Input: part model. Units: mm. Frame: model coordinates. A direction names the side the tool comes from. Coordinates: 2 decimals unless noted, no trailing zeros. Write each loop counter-clockwise with the first axis right and the second up, starting at its lowest first coordinate (ties: lowest second). Pieces come first, ordered by that corner, then holes. Notation, with made-up numbers: (-35.75, 19) -> (-31.75, 19) arc R29 ccw to (-31.75, 50) -> close; hole circle Ø4 at (-15, -31.5). An arc over 180 degrees is marked (long way). Use one line per item in the form item = value. Start each with the question number.
(1) Set-up query: faces 1 (the face through (-51, -7.62, 3)), 2 (the face through (-0.486, -91.437, 0.715)), 3 (the face through (13, -25, 3.175)). Return all of +Z, -Z, +X, -X, +Y, -Y with unobstructed straight access to the full face (end or side cutting, diameter ignored); none if empty.
(2) Pull-direction query (Y, two-part tool) for faces 4 (the face through (13, 19, 3.175)), 5 (the face through (-69.85, 0, 1)), 6 (the face through (-68.604, 32.175, 0.715)); classes: released by +Y, released by -Y, zero draft, split by the parting line, or undercut.
(3) Cut plane B-B on x = 12.7. State how many separate pieces and enclosed holes the cut face has, plus the area to 3 significant figures.
(4) Cut plane A-A on y = 0. Return the cut outline in (x, z) (3 decimals).
(5) First-contact query: pin 1 (3 mm diameter, centred on x = -44.5, y = 1, fed in from -Z); pin 2 (9 mm diameter, centred on x = -25.4, y = 0, fed in from -Z) (3 decimals); pin 3 (5 mm diameter, centred on x = -18, z = 3, fed in from +Y). Flat tips, straight axial feed; report the tip coordinate or a pass-through.
(6) Ray query, line 1 along Y through (x, z) = (0, 2) (3 decimals); line 2 along Y through (x, z) = (12.5, 2.25); line 3 along Z through (x, y) = (-30.5, 22). Return the intervals inside material, ascending.
(7) Cut plane C-C on y = -50.8. Return the cut outline in (x, z) (3 decimals), plus the area to 3 significant figures.
```python
from build123d import *

# Parameters (mm, degrees)
F2_R     = 2.3876
F2_R_2   = 2.794
F2_R_3   = 1.3
F3_DEPTH = 6.35
F4_R     = 6.5
F5_DEPTH = 3.175
F7_DEPTH = 5.08
F8_R     = 15.875
F9_DEPTH = 25.4


with BuildPart() as f3:
    # F2 (on Top) → F3 (new body)
    with BuildSketch(Plane.XY):
        with BuildLine():
            ThreePointArc((30.6280254128, -77.5120508256), (38.0547799414, -65.063355973), (40.64, -50.8))
            ThreePointArc((40.64, -50.8), (-14.263355973, -12.7452200586), (-30.6280254128, -77.5120508256))
            ThreePointArc((-30.6280254128, -77.5120508256), (0, -91.44), (30.6280254128, -77.5120508256))
        make_face()
        with Locations((-28.596158833, -67.31)):
            Circle(F2_R, mode=Mode.SUBTRACT)
        with Locations((28.596158833, -67.31)):
            Circle(F2_R, mode=Mode.SUBTRACT)
        with Locations((0, -17.78)):
            Circle(F2_R, mode=Mode.SUBTRACT)
        with Locations((12.7, -21.9970452561)):
            Circle(F2_R_2, mode=Mode.SUBTRACT)
        with BuildLine():
            ThreePointArc((-30.6280254128, -77.5120508256), (-14.263355973, -12.7452200586), (40.64, -50.8))
            ThreePointArc((40.64, -50.8), (38.0547799414, -65.063355973), (30.6280254128, -77.5120508256))
            Line((30.6280254128, -77.5120508256), (65.1568869123, -37.9212738245))
            ThreePointArc((65.1568869123, -37.9212738245), (68.6381780975, -32.0859481123), (69.85, -25.4))
            Line((69.85, -25.4), (69.85, 25.4))
            ThreePointArc((69.85, 25.4), (68.6381780975, 32.0859481123), (65.1568869123, 37.9212738245))
            Line((65.1568869123, 37.9212738245), (30.6280254128, 77.5120508256))
            ThreePointArc((30.6280254128, 77.5120508256), (38.0547799414, 65.063355973), (40.64, 50.8))
            ThreePointArc((40.64, 50.8), (-14.263355973, 12.7452200586), (-30.6280254128, 77.5120508256))
            Line((-30.6280254128, 77.5120508256), (-65.1568869123, 37.9212738245))
            ThreePointArc((-65.1568869123, 37.9212738245), (-68.6381780975, 32.0859481123), (-69.85, 25.4))
            Line((-69.85, 25.4), (-69.85, 0))
            Line((-69.85, 0), (-69.85, -25.4))
            ThreePointArc((-69.85, -25.4), (-68.6381780975, -32.0859481123), (-65.1568869123, -37.9212738245))
            Line((-65.1568869123, -37.9212738245), (-30.6280254128, -77.5120508256))
        make_face()
        with Locations((-56.8621778265, -28.9)):
            Circle(F2_R_3, mode=Mode.SUBTRACT)
        with Locations((-44.7378221735, -28.9)):
            Circle(F2_R_3, mode=Mode.SUBTRACT)
        with Locations((-50.8, -18.4)):
            Circle(F2_R_3, mode=Mode.SUBTRACT)
        with Locations((44.7378221735, -28.9)):
            Circle(F2_R_3, mode=Mode.SUBTRACT)
        with Locations((56.8621778265, -28.9)):
            Circle(F2_R_3, mode=Mode.SUBTRACT)
        with Locations((50.8, -18.4)):
            Circle(F2_R_3, mode=Mode.SUBTRACT)
        with Locations((-56.8621778265, 21.9)):
            Circle(F2_R_3, mode=Mode.SUBTRACT)
        with Locations((-44.7378221735, 21.9)):
            Circle(F2_R_3, mode=Mode.SUBTRACT)
        with Locations((-50.8, 32.4)):
            Circle(F2_R_3, mode=Mode.SUBTRACT)
        with Locations((-25.4, 0)):
            Circle(F2_R_2, mode=Mode.SUBTRACT)
        with Locations((44.7378221735, 21.9)):
            Circle(F2_R_3, mode=Mode.SUBTRACT)
        with Locations((56.8621778265, 21.9)):
            Circle(F2_R_3, mode=Mode.SUBTRACT)
        with Locations((50.8, 32.4)):
            Circle(F2_R_3, mode=Mode.SUBTRACT)
        with BuildLine():
            ThreePointArc((40.64, 50.8), (38.0547799414, 65.063355973), (30.6280254128, 77.5120508256))
            ThreePointArc((30.6280254128, 77.5120508256), (0, 91.44), (-30.6280254128, 77.5120508256))
            ThreePointArc((-30.6280254128, 77.5120508256), (-14.263355973, 12.7452200586), (40.64, 50.8))
        make_face()
        with Locations((-28.596158833, 67.31)):
            Circle(F2_R, mode=Mode.SUBTRACT)
        with Locations((0, 17.78)):
            Circle(F2_R, mode=Mode.SUBTRACT)
        with Locations((12.7, 21.9970452561)):
            Circle(F2_R_2, mode=Mode.SUBTRACT)
        with Locations((28.596158833, 67.31)):
            Circle(F2_R, mode=Mode.SUBTRACT)
    extrude(amount=F3_DEPTH)

    # F4 (on Top) → F5 (cut)
    with BuildSketch(Plane.XY):
        with Locations((-25.4, 0)):
            Circle(F4_R)
        with Locations((12.7, 21.9970452561)):
            Circle(F4_R)
        with Locations((12.7, -21.9970452561)):
            Circle(F4_R)
    extrude(amount=F5_DEPTH, mode=Mode.SUBTRACT)

    # F6 (on Top) → F7 (join)
    with BuildSketch(Plane.XY):
        with BuildLine():
            ThreePointArc((-69.85, -25.4), (-68.6381780975, -32.0859481123), (-65.1568869123, -37.9212738245))
            Line((-65.1568869123, -37.9212738245), (-30.6280254128, -77.5120508256))
            ThreePointArc((-30.6280254128, -77.5120508256), (0, -91.44), (30.6280254128, -77.5120508256))
            Line((30.6280254128, -77.5120508256), (65.1568869123, -37.9212738245))
            ThreePointArc((65.1568869123, -37.9212738245), (68.6381780975, -32.0859481123), (69.85, -25.4))
            Line((69.85, -25.4), (69.85, 25.4))
            ThreePointArc((69.85, 25.4), (68.6381780975, 32.0859481123), (65.1568869123, 37.9212738245))
            Line((65.1568869123, 37.9212738245), (30.6280254128, 77.5120508256))
            ThreePointArc((30.6280254128, 77.5120508256), (0, 91.44), (-30.6280254128, 77.5120508256))
            Line((-30.6280254128, 77.5120508256), (-65.1568869123, 37.9212738245))
            ThreePointArc((-65.1568869123, 37.9212738245), (-68.6381780975, 32.0859481123), (-69.85, 25.4))
            Line((-69.85, 25.4), (-69.85, -25.4))
        make_face()
        with BuildLine():
            Line((-28.7137738245, -75.842547649), (-63.242635324, -36.2517706479))
            ThreePointArc((-63.242635324, -36.2517706479), (-66.2597543512, -31.194488364), (-67.31, -25.4))
            Line((-67.31, -25.4), (-67.31, 25.4))
            ThreePointArc((-67.31, 25.4), (-66.2597543512, 31.194488364), (-63.242635324, 36.2517706479))
            Line((-63.242635324, 36.2517706479), (-28.7137738245, 75.842547649))
            ThreePointArc((-28.7137738245, 75.842547649), (0, 88.9), (28.7137738245, 75.842547649))
            Line((28.7137738245, 75.842547649), (63.242635324, 36.2517706479))
            ThreePointArc((63.242635324, 36.2517706479), (66.2597543512, 31.194488364), (67.31, 25.4))
            Line((67.31, 25.4), (67.31, -25.4))
            ThreePointArc((67.31, -25.4), (66.2597543512, -31.194488364), (63.242635324, -36.2517706479))
            Line((63.242635324, -36.2517706479), (28.7137738245, -75.842547649))
            ThreePointArc((28.7137738245, -75.842547649), (0, -88.9), (-28.7137738245, -75.842547649))
        make_face(mode=Mode.SUBTRACT)
    extrude(amount=-F7_DEPTH)

    # F8 (on Top) → F9 (cut)
    with BuildSketch(Plane.XY):
        with Locations((0, -50.8)):
            Circle(F8_R)
        with Locations((0, 50.8)):
            Circle(F8_R)
        with BuildLine():
            ThreePointArc((-43.18, 5.588), (-43.7751590206, 7.0248409794), (-45.212, 7.62))
            Line((-45.212, 7.62), (-56.388, 7.62))
            ThreePointArc((-56.388, 7.62), (-57.8248409794, 7.0248409794), (-58.42, 5.588))
            Line((-58.42, 5.588), (-58.42, -5.588))
            ThreePointArc((-58.42, -5.588), (-57.8248409794, -7.0248409794), (-56.388, -7.62))
            Line((-56.388, -7.62), (-45.212, -7.62))
            ThreePointArc((-45.212, -7.62), (-43.7751590206, -7.0248409794), (-43.18, -5.588))
            Line((-43.18, -5.588), (-43.18, 5.588))
        make_face()
        with BuildLine():
            ThreePointArc((58.42, 5.588), (57.8248409794, 7.0248409794), (56.388, 7.62))
            Line((56.388, 7.62), (45.212, 7.62))
            ThreePointArc((45.212, 7.62), (43.7751590206, 7.0248409794), (43.18, 5.588))
            Line((43.18, 5.588), (43.18, -5.588))
            ThreePointArc((43.18, -5.588), (43.7751590206, -7.0248409794), (45.212, -7.62))
            Line((45.212, -7.62), (56.388, -7.62))
            ThreePointArc((56.388, -7.62), (57.8248409794, -7.0248409794), (58.42, -5.588))
            Line((58.42, -5.588), (58.42, 5.588))
        make_face()
    extrude(amount=F9_DEPTH, mode=Mode.SUBTRACT)


solid = f3.part
```
Values:
q1.face_1 = +Z, -Z
q1.face_2 = +Z, -Z, -Y
q1.face_3 = -Z
q2.face_4 = undercut
q2.face_5 = zero draft
q2.face_6 = released by +Y
q3.separate_pieces = 5
q3.enclosed_holes = 0
q3.area = 803 mm2
q4.outline = (-69.85, -5.08) -> (-67.31, -5.08) -> (-67.31, 0) -> (-58.42, 0) -> (-58.42, 6.35) -> (-69.85, 6.35) -> close; (-43.18, 0) -> (-31.9, 0) -> (-31.9, 3.175) -> (-28.194, 3.175) -> (-28.194, 6.35) -> (-43.18, 6.35) -> close; (-22.606, 3.175) -> (-18.9, 3.175) -> (-18.9, 0) -> (43.18, 0) -> (43.18, 6.35) -> (-22.606, 6.35) -> close; (58.42, 0) -> (67.31, 0) -> (67.31, -5.08) -> (69.85, -5.08) -> (69.85, 6.35) -> (58.42, 6.35) -> close
q5.pin_1 = 0
q5.pin_2 = 3.175
q5.pin_3 = 88.37
q6.line_1 = -91.44 to -66.675, -34.925 to -20.168, -15.392 to 15.392, 20.168 to 34.925, 66.675 to 91.44
q6.line_2 = -89.47 to -60.59, -41.01 to -28.49, -15.5 to 15.5, 28.49 to 41.01, 60.59 to 89.47
q6.line_3 = 0 to 6.35
q7.outline = (-53.925, -5.08) -> (-50.554, -5.08) -> (-50.554, 0) -> (-15.875, 0) -> (-15.875, 6.35) -> (-53.925, 6.35) -> close; (15.875, 0) -> (50.554, 0) -> (50.554, -5.08) -> (53.925, -5.08) -> (53.925, 6.35) -> (15.875, 6.35) -> close
q7.area = 517 mm2
